```python
from build123d import *

# Parameters (mm, degrees)
SKETCH1_W               = 44
SKETCH1_H               = 20
BOSS_EXTRUDE1_DEPTH     = 21.2
CUT_EXTRUDE1_DEPTH      = 32.771685508
CUT_EXTRUDE1_DEPTH_BACK = 32.771685508
SKETCH4_W               = 17
SKETCH4_H               = 15
CUT_EXTRUDE3_DEPTH      = 0.7
CHAMFER3_SIZE           = 0.7
CHAMFER4_SIZE           = 0.7
SKETCH5_W               = 7.5
SKETCH5_H               = 1.5
CUT_EXTRUDE4_DEPTH      = 33.147161617


with BuildPart() as part:
    # Sketch1 → Boss-Extrude1 (new body)
    with BuildSketch(Plane.XY):
        Rectangle(SKETCH1_W, SKETCH1_H)
    extrude(amount=BOSS_EXTRUDE1_DEPTH)

    # Sketch2 → Cut-Extrude1 (cut, two sides: drawn at the far end of the back side and taken through both)
    with BuildSketch(Plane(origin=(0, -10, 11.2), x_dir=(1, 0, 0), z_dir=(0, 1, 0)).offset(-CUT_EXTRUDE1_DEPTH_BACK)):
        Polygon((-89.868081564, -89.441697876), (-22, -8), (-6, 11.2), (61.868081564, 92.641697876), (-101.015314189, 228.377861004), (-252.751477317, 46.294465251), align=None)
    extrude(amount=CUT_EXTRUDE1_DEPTH + CUT_EXTRUDE1_DEPTH_BACK, mode=Mode.SUBTRACT)

    # Sketch4 → Cut-Extrude3 (cut)
    with BuildSketch(Plane(origin=(-3.540983607, 0, -2.950819672), x_dir=(-0.6401843996644798, 0, 0.7682212795973761), z_dir=(-0.7682212795973761, 0, -0.6401843996644798))):
        with Locations((14.841106398, 0)):
            Rectangle(SKETCH4_W, SKETCH4_H)
    extrude(amount=-CUT_EXTRUDE3_DEPTH, mode=Mode.SUBTRACT)

    # Chamfer3
    chamfer3_edges = [part.edges().sort_by_distance(p)[0] for p in [
        (-13.042028396, 7.5, 8.450434076),
        (-13.042028396, -7.5, 8.450434076),
        (-7.600460999, 0, 1.920553199),
    ]]
    chamfer(chamfer3_edges, length=CHAMFER3_SIZE - 0.0001)  # a hair under: the kernel refuses the full size

    # Chamfer4
    chamfer4_edges = [part.edges().sort_by_distance(p)[0] for p in [
        (-17.945840898, 0, 15.428444032),
    ]]
    chamfer(chamfer4_edges, length=CHAMFER4_SIZE - 0.0001)  # a hair under: the kernel refuses the full size

    # Sketch5 → Cut-Extrude4 (cut, through all)
    with BuildSketch(Plane(origin=(0, 0, 0), x_dir=(-1, 0, 0), z_dir=(0, 0, -1))):
        with Locations((-4.35, 9.25)):
            Rectangle(SKETCH5_W, SKETCH5_H)
        with Locations((-4.35, -9.25)):
            Rectangle(SKETCH5_W, SKETCH5_H)
    extrude(amount=-CUT_EXTRUDE4_DEPTH, mode=Mode.SUBTRACT)


solid = part.part
```
Geometry: final body of the model. Coordinates: model frame, mm. A direction names the side the tool comes from. Round coordinates to 2 decimals unless told otherwise and drop trailing zeros. Loops run counter-clockwise (first coordinate to the right, second up) from the corner with the lowest first, then second, coordinate; pieces in that order, holes last.
Item 1: Line query: L1, parallel to X at y = -8.75, z = 3.25; L2, parallel to Y at x = 6, z = 2.25; L3, parallel to X at y = 9, z = 5.25 (3 decimals). Output: solid intervals per line, ascending.
Checked values:
L1: x = -8.71 to 0.6, 8.1 to 22
L2: y = -8.5 to 8.5
L3: x = -10.375 to 0.6, 8.1 to 22
Item 2: Mould query, pull axis X, two halves, no side actions, for faces 1 (the flat face through (4, 8.5, 10)), 2 (the flat face through (-12.207, 0.105, 8.542)), 3 (the flat face through (0.6, -9, 10)), 4 (the flat face through (-8, 10, 13)). Classes: released by +X, released by -X, zero draft, split by the parting line, or undercut.
Checked values:
face 1: undercut
face 2: released by -X
face 3: undercut
face 4: zero draft
Item 3: Section D-D, the plane z = 16.75. Output: boundary loops of the cut face in (x, y), plus the area to 3 significant figures.
Checked values:
outline: (-19.96, -10) - (0.6, -10) - (0.6, -8.5) - (8.1, -8.5) - (8.1, -10) - (22, -10) - (22, 10) - (8.1, 10) - (8.1, 8.5) - (0.6, 8.5) - (0.6, 10) - (-19.96, 10) - close
area: 817 mm2
Item 4: Reachability of faces 5 (the flat face through (-17.998, -0.115, 14.936)), 6 (the flat face through (4, -8.5, 10)), 7 (the flat face through (8.1, 9, 10)), 8 (the flat face through (-7.107, -0.115, 1.883)) from +Z, -Z, +X, -X, +Y, -Y: full face, straight path, thin tool, end or side. Return the list, or none.
Checked values:
face 5: -Z, -X
face 6: +Z, -Z, -Y
face 7: +Z, -Z, +Y
face 8: -X
Item 5: Contact query for flat-ended pins moving along their axis: P1, Ø2, axis at x = 3, z = 12.5, coming from the -Y side; P2, Ø3, axis at y = 0, z = 14, coming from the -X side; P3, Ø1.2, axis at y = -9.5, z = 6.5, coming from the -X side; P4, Ø8, axis at x = -12, z = 7, coming from the +Y side. Output: stop coordinate, or through.
Checked values:
P1: stops at y = -8.5
P2: stops at x = -18.92
P3: stops at x = -11.92
P4: stops at y = 10
Item 6: Section C-C, the plane x = 3. Output: boundary loops of the cut face in (y, z).
Checked values:
outline: (-8.5, 0) - (8.5, 0) - (8.5, 21.2) - (-8.5, 21.2) - close
